Source: CAD feature listing. Evaluate the final solid. Frame: model axes, mm. A direction names the side the tool comes from. Give positions to 0.01 mm unless a question says otherwise; leave off trailing zeros. Loops run counter-clockwise (first coordinate to the right, second up) from the corner with the lowest first, then second, coordinate; pieces in that order, holes last. Notation, with made-up numbers: M 67,-30.75 L 91,-30.75 A15 cw 91,-11.75 Z; hole C 16.25,75 d5. An arc over 180 degrees is marked long. Put each result on its own line as item: value.
from build123d import *

# Parameters (mm, degrees)
SKETCH_W      = 28
SKETCH_H      = 28
SKETCH_R      = 1.75
SKETCH_R_2    = 1.25
PAD_DEPTH     = 3
SKETCH001_R   = 3.5
SKETCH001_R_2 = 1.25
PAD001_DEPTH  = 2
FILLET_R      = 3


with BuildPart() as part:
    # Sketch → Pad (new body)
    with BuildSketch(Plane.XY):
        with Locations((14, 14)):
            Rectangle(SKETCH_W, SKETCH_H)
        with Locations((4, 24)):
            Circle(SKETCH_R, mode=Mode.SUBTRACT)
        with Locations((24, 24)):
            Circle(SKETCH_R_2, mode=Mode.SUBTRACT)
        with Locations((24, 4)):
            Circle(SKETCH_R_2, mode=Mode.SUBTRACT)
        with Locations((4, 4)):
            Circle(SKETCH_R, mode=Mode.SUBTRACT)
    extrude(amount=PAD_DEPTH)

    # Sketch001 (on Face10 of Pad) → Pad001 (join)
    with BuildSketch(Plane.XY.offset(3)):
        with Locations((24, 4)):
            Circle(SKETCH001_R)
        with Locations((24, 4)):
            Circle(SKETCH001_R_2, mode=Mode.SUBTRACT)
        with Locations((24, 24)):
            Circle(SKETCH001_R)
        with Locations((24, 24)):
            Circle(SKETCH001_R_2, mode=Mode.SUBTRACT)
    extrude(amount=PAD001_DEPTH)

    # Fillet
    fillet_edges = [part.edges().sort_by_distance(p)[0] for p in [
        (0, 0, 1.5),
        (0, 28, 1.5),
        (28, 0, 1.5),
        (28, 28, 1.5),
    ]]
    fillet(fillet_edges, radius=FILLET_R)


solid = part.part
1. Material intervals for line 1 (Y direction, x = 24, z = 1.85); line 2 (Y direction, x = 24, z = 3.05); line 3 (Y direction, x = 4, z = 0.8), sorted ascending. Write a range as from..to.
Found:
line 1: 0..2.75, 5.25..22.75, 25.25..28
line 2: 0.5..2.75, 5.25..7.5, 20.5..22.75, 25.25..27.5
line 3: 0..2.25, 5.75..22.25, 25.75..28
2. Section query A-A (x = 24). Output: boundary loops of the cut face in (y, z).
Found:
outline: M 0,0 L 2.75,0 L 2.75,5 L 0.5,5 L 0.5,3 L 0,3 Z; M 5.25,0 L 22.75,0 L 22.75,5 L 20.5,5 L 20.5,3 L 7.5,3 L 7.5,5 L 5.25,5 Z; M 25.25,0 L 28,0 L 28,3 L 27.5,3 L 27.5,5 L 25.25,5 Z
3. Draft query along Y for faces 3 (the cylindrical face through (3.772, 25.735, 1.479)), 4 (the flat face through (0, 14, 1)), 5 (the cylindrical face through (25.155, 23.521, 2.465)), 6 (the cylindrical face through (0.9, 0.86, 1.52)). Return one class per face: pulls with the +Y half, pulls with the -Y half, needs draft (parallel to the pull), parting line crosses it, or undercut.
Found:
face 3: undercut
face 4: needs draft
face 5: undercut
face 6: pulls with the -Y half
4. Access query for faces 1 (the cylindrical face through (27.34, 25.05, 3.99)), 2 (the cylindrical face through (2.25, 4.08, 1.48)). Directions: +Z, -Z, +X, -X, +Y, -Y. A direction counts if a zero-diameter tool reaches every point of the face in a straight line with its end or side. Return the directions, or none.
Found:
face 1: +Z
face 2: +Z, -Z
5. Contact query for flat-ended pins moving along their axis: P1, Ø4.5, axis at x = 4, y = 24, coming from the +Z side; P2, Ø2, axis at x = 24, y = 24, coming from the -Z side (1 decimal). Output: stop coordinate, or through.
Found:
P1: z = 3
P2: through
6. Section query B-B (z = 2.6). Output: boundary loops of the cut face in (x, y), plus the area to 3 significant figures.
Found:
outline: M 0,3 A3 ccw 3,0 L 25,0 A3 ccw 28,3 L 28,25 A3 ccw 25,28 L 3,28 A3 ccw 0,25 Z; hole C 4,4 d3.5; hole C 4,24 d3.5; hole C 24,4 d2.5; hole C 24,24 d2.5
area: 747 mm^2
7. Section query D-D (x = 4). Output: boundary loops of the cut face in (y, z).
Found:
outline: M 0,0 L 2.25,0 L 2.25,3 L 0,3 Z; M 5.75,0 L 22.25,0 L 22.25,3 L 5.75,3 Z; M 25.75,0 L 28,0 L 28,3 L 25.75,3 Z
8. Section query C-C (y = 4). Output: boundary loops of the cut face in (x, z).
Found:
outline: M 0,0 L 2.25,0 L 2.25,3 L 0,3 Z; M 5.75,0 L 22.75,0 L 22.75,5 L 20.5,5 L 20.5,3 L 5.75,3 Z; M 25.25,0 L 28,0 L 28,3 L 27.5,3 L 27.5,5 L 25.25,5 Z
